Geometry check sheet. Reference: drawing and pictorial views, mm from the part's lowest x, y, z. A direction names the side the tool comes from. Give positions to 0.01 mm unless a question says otherwise; leave off trailing zeros. One line per item, written item: value. Start each with the question number.
1. Release check for a two-part mould opening along Z. For the marked faces 3, 4 and 5 record: pulls with the +Z half, pulls with the -Z half, needs draft (parallel to the pull), parting line crosses it, or undercut.
2. Scan lines: line 1 (Z direction, x = 3.45, y = 3.55); line 2 (Z direction, x = 3.25, y = 1.05) (1 decimal); line 3 (X direction, y = 3.6, z = 5.5) (1 decimal). Record each from-to range of solid material in increasing order.
3. Gauge pin test, flat end, axial feed: pin 1 (1 mm diameter, centred on x = 2, y = 1, fed in from -Z). Record the tip position at first contact, or that the pin passes through.
4. Tool access check on the marked faces 1 and 2. Record the directions out of +Z, -Z, +X, -X, +Y, -Y that give a thin tool (end or side, any length) a straight path to the whole face; none if there is none.
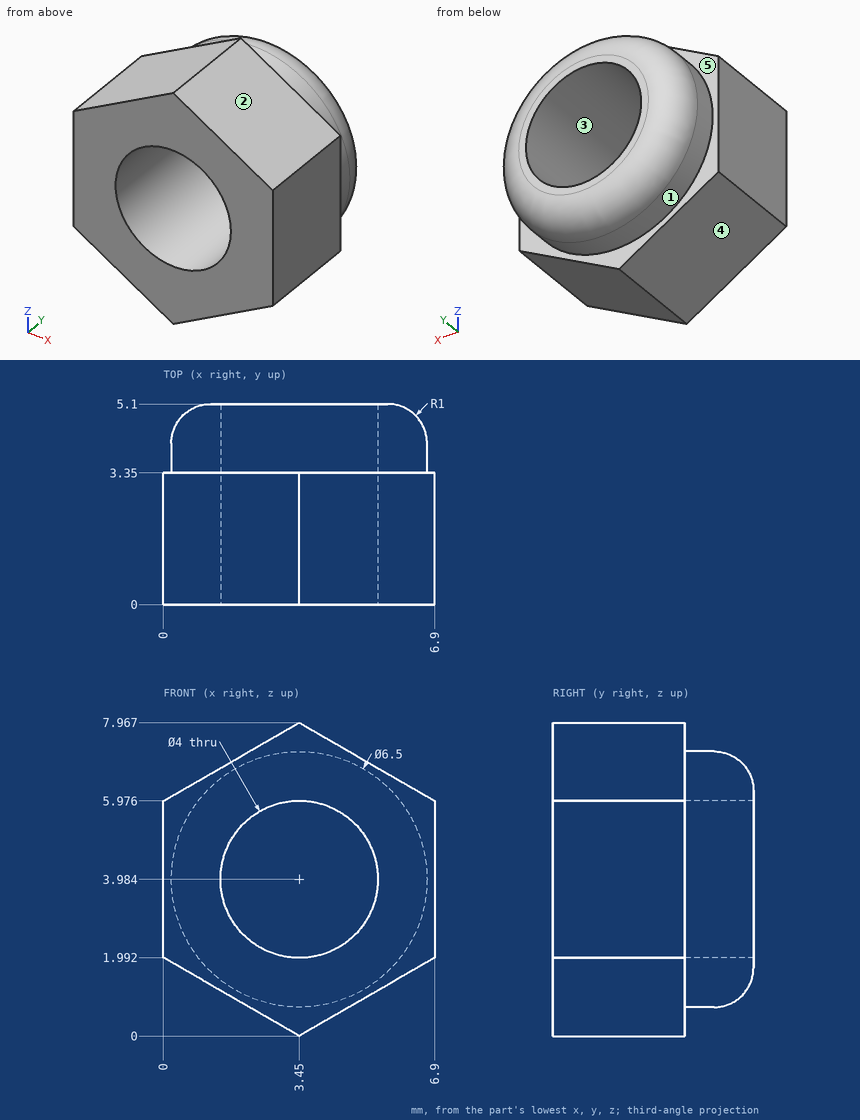
Report:
1. face 3: undercut
1. face 4: pulls with the -Z half
1. face 5: needs draft
2. line 1: z = 0.73 to 1.98, 5.98 to 7.23
2. line 2: z = 0.1 to 2, 6 to 7.9
2. line 3: x = 0.6 to 2.1, 4.8 to 6.3
3. pin 1: stops at z = 0.55
4. face 1: +Y
4. face 2: +Z, +X, +Y, -Y
